from build123d import *

# Parameters (mm, degrees)
BOSS_EXTRUDE1_DEPTH = 50
BOSS_EXTRUDE2_DEPTH = 35
SKETCH4_R           = 2.2
CUT_EXTRUDE1_DEPTH  = 35
SKETCH5_R           = 4
CUT_EXTRUDE2_DEPTH  = 5
SKETCH6_R           = 4
CUT_EXTRUDE3_DEPTH  = 34
SKETCH7_R           = 4
SKETCH7_R_2         = 2.2
BOSS_EXTRUDE3_DEPTH = 8
SKETCH8_W           = 72
SKETCH8_H           = 52
BOSS_EXTRUDE4_DEPTH = 10
FILLET1_R           = 5
CUT_EXTRUDE5_DEPTH  = 28
SKETCH11_R          = 11.145843878
SKETCH11_R_2        = 4
BOSS_EXTRUDE6_DEPTH = 3


with BuildPart() as part:
    # Sketch1 → Boss-Extrude1 (new body)
    with BuildSketch(Plane(origin=(0, 0, 0), x_dir=(1, 0, 0), z_dir=(0, 1, 0))):
        with BuildLine():
            Line((-28, 23.5), (-28, -8.5))
            ThreePointArc((-28, -8.5), (-24.485281374, -16.985281374), (-16, -20.5))
            Line((-16, -20.5), (16, -20.5))
            ThreePointArc((16, -20.5), (24.485281374, -16.985281374), (28, -8.5))
            Line((28, -8.5), (28, 23.5))
            Line((28, 23.5), (36, 23.5))
            Line((36, 23.5), (36, 15.5))
            Line((36, 15.5), (36, -8.5))
            Line((36, -8.5), (36, -28.5))
            Line((36, -28.5), (16, -28.5))
            Line((16, -28.5), (-16, -28.5))
            Line((-16, -28.5), (-36, -28.5))
            Line((-36, -28.5), (-36, -8.5))
            Line((-36, -8.5), (-36, 15.5))
            Line((-36, 15.5), (-36, 23.5))
            Line((-36, 23.5), (-28, 23.5))
        make_face()
    extrude(amount=BOSS_EXTRUDE1_DEPTH)

    # Sketch3 → Boss-Extrude2 (add)
    with BuildSketch(Plane(origin=(0, 50, 0), x_dir=(1, 0, 0), z_dir=(0, 1, 0))):
        with BuildLine():
            Line((-36, 7.5), (-36, -8.5))
            Line((-36, -8.5), (-36, -28.5))
            Line((-36, -28.5), (-16, -28.5))
            Line((-16, -28.5), (16, -28.5))
            Line((16, -28.5), (36, -28.5))
            Line((36, -28.5), (36, -8.5))
            Line((36, -8.5), (36, 7.5))
            Line((36, 7.5), (28, 7.5))
            Line((28, 7.5), (21.128428342, 7.5))
            ThreePointArc((21.128428342, 7.5), (0.128823476, -13.371176524), (-20.87078139, 7.5))
            Line((-20.87078139, 7.5), (-28, 7.5))
            Line((-28, 7.5), (-36, 7.5))
        make_face()
    extrude(amount=BOSS_EXTRUDE2_DEPTH)

    # Sketch4 → Cut-Extrude1 (cut)
    with BuildSketch(Plane(origin=(0, 0, 20.5), x_dir=(-1, 0, 0), z_dir=(0, 0, -1))):
        with Locations((8, 33)):
            Circle(SKETCH4_R)
        with Locations((-8, 33)):
            Circle(SKETCH4_R)
        with Locations((-8, 17)):
            Circle(SKETCH4_R)
        with Locations((8, 17)):
            Circle(SKETCH4_R)
    extrude(amount=-CUT_EXTRUDE1_DEPTH, mode=Mode.SUBTRACT)

    # Sketch5 → Cut-Extrude2 (cut)
    with BuildSketch(Plane(origin=(0, 0, 20.5), x_dir=(-1, 0, 0), z_dir=(0, 0, -1))):
        with Locations((-8, 17)):
            Circle(SKETCH5_R)
        with Locations((8, 17)):
            Circle(SKETCH5_R)
    extrude(amount=-CUT_EXTRUDE2_DEPTH, mode=Mode.SUBTRACT)

    # Sketch6 → Cut-Extrude3 (cut)
    with BuildSketch(Plane.XY.offset(28.5)):
        with Locations((-8, 68)):
            Circle(SKETCH6_R)
        with Locations((8, 68)):
            Circle(SKETCH6_R)
    extrude(amount=-CUT_EXTRUDE3_DEPTH, mode=Mode.SUBTRACT)

    # Sketch7 → Boss-Extrude3 (add)
    # profile 1 of 2: a face of its own
    with BuildSketch(Plane.XY.offset(28.5)):
        with Locations((-8, 68)):
            Circle(SKETCH7_R)
        with Locations((-8, 68)):
            Circle(SKETCH7_R_2, mode=Mode.SUBTRACT)
    # profile 2 of 2: a face of its own
    with BuildSketch(Plane.XY.offset(28.5)):
        with Locations((8, 68)):
            Circle(SKETCH7_R)
        with Locations((8, 68)):
            Circle(SKETCH7_R_2, mode=Mode.SUBTRACT)
    extrude(amount=-BOSS_EXTRUDE3_DEPTH)

    # Sketch8 → Boss-Extrude4 (add)
    with BuildSketch(Plane.XZ):
        with Locations((0, 2.5)):
            Rectangle(SKETCH8_W, SKETCH8_H)
    extrude(amount=BOSS_EXTRUDE4_DEPTH)

    # Fillet1
    fillet1_edges = [part.edges().sort_by_distance(p)[0] for p in [
        (-36, -10, 2.5),
        (36, -10, 2.5),
        (32, 50, -23.5),
        (32, 50, -7.5),
        (-32, 50, -23.5),
        (-32, 50, -7.5),
    ]]
    fillet(fillet1_edges, radius=FILLET1_R)

    # Sketch9 → Cut-Extrude5 (cut)
    with BuildSketch(Plane.XZ.offset(10)):
        Polygon((-3.635500279, -0.98), (-7.399824034, -7.5), (7.657470986, -7.5), (3.893147231, -0.98), align=None)
        Polygon((7.657470986, -7.5), (-7.399824034, -7.5), (-3.635500279, -14.02), (3.893147231, -14.02), align=None)
    extrude(amount=-CUT_EXTRUDE5_DEPTH, mode=Mode.SUBTRACT)

    # Sketch11 → Boss-Extrude6 (add)
    with BuildSketch(Plane(origin=(0, -10, 0), x_dir=(-1, 0, 0), z_dir=(0, -1, 0))):
        with Locations((-0.128823476, 7.5)):
            Circle(SKETCH11_R)
        with Locations(Location((-0.128823476, 7.5, 0), (0, 0, 90))):
            Circle(SKETCH11_R_2, mode=Mode.SUBTRACT)
    extrude(amount=-BOSS_EXTRUDE6_DEPTH)


solid = part.part
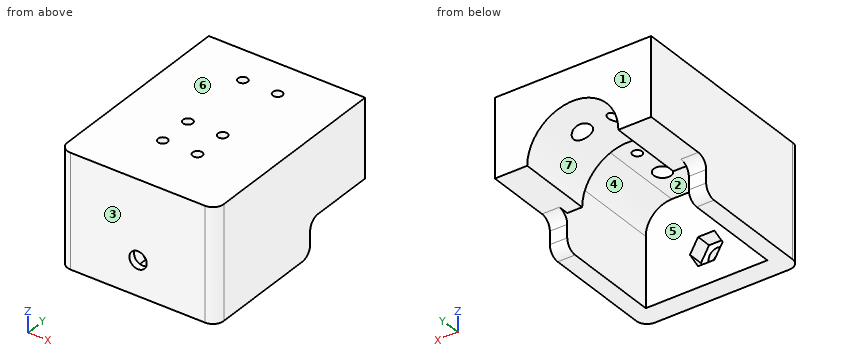
Design review of the part built by this model. Coordinates are the model's own, in mm. Face numbers are marked on the shaded views. A direction names the side the tool comes from. Give positions to 0.01 mm unless a question says otherwise; leave off trailing zeros. Loops run counter-clockwise (first coordinate to the right, second up) from the corner with the lowest first, then second, coordinate; pieces in that order, holes last. Notation, with made-up numbers: M 57,54.5 L 110,54.5 A17 cw 110,84.5 Z; hole C 45,-0.5 d8. An arc over 180 degrees is marked long. One line per question, with ' | ' between items. Start each with the question number.
1. Add section D-D (z = 11). Write out the cut boundary in (x, y), plus the area to 3 significant figures.
2. Add section C-C (x = -29.5). Write out the cut boundary in (y, z).
3. To check wall thickness, follow L1, parallel to Y at x = -8, z = 26.5; L2, parallel to X at y = 10, z = -16; L3, parallel to Y at x = 8, z = 22.15. State the ranges of each line that lie inside material, in increasing order.
4. The part is to be moulded in two halves that separate along Y. For the marked faces 1, 2, 3 and 4, say which applies: released by +Y, released by -Y, zero draft, split by the parting line, or undercut.
5. Add section A-A (y = 17). Write out the cut boundary in (x, z), plus the area to 3 significant figures.
6. Add section B-B (y = 28.5). Write out the cut boundary in (x, z), plus the area to 3 significant figures.
7. For the marked faces 5, 6 and 7, list the 3-axis set-ups (+Z, -Z, +X, -X, +Y, -Y) from which the entire face can be reached by the end or side of a thin tool; tool diameter is ignored.
8. Insertion check: P1, Ø16.5, axis at x = 29, y = 67.5, coming from the -Z side; P2, Ø1.5, axis at x = -15.5, y = 31, coming from the -Z side; P3, Ø7, axis at x = 0.13, z = -7.5, coming from the +Y side; P4, Ø13, axis at x = -7, z = -3, coming from the +Y side. Each pin has a flat end and moves straight along its axis. Give the tip position at first contact, or say it passes through.
Worked out:
1) outline: M -36,-5 A5 ccw -31,-10 L 31,-10 A5 ccw 36,-5 L 36,85 L 9.82,85 L 9.82,71.56 A4 cw 9.82,64.44 L 9.82,50 L 27.74,50 L 27.74,0 L -27.74,0 L -27.74,50 L -9.56,50 L -9.56,64.32 A4 cw -9.56,71.68 L -9.56,85 L -36,85 Z | area: 3,350 mm²
2) outline: M -10,-23.5 L 45,-23.5 A5 ccw 50,-18.5 L 50,-12.5 A5 cw 55,-7.5 L 85,-7.5 L 85,28.5 L -10,28.5 Z
3) L1: y = -10 to 14.8, 19.2 to 30.8, 35.2 to 65.8, 70.2 to 85 | L2: x = -36 to -28, 28 to 36 | L3: y = -10 to 13, 21 to 30.8, 35.2 to 65.8, 70.2 to 85
4) face 1: released by +Y | face 2: undercut | face 3: released by -Y | face 4: undercut
5) outline: M -36,-23.5 L -28,-23.5 L -28,8.5 A12 cw -16,20.5 L -12,20.5 L -12,25.5 L -10.2,25.5 L -10.2,28.5 L -36,28.5 Z; M -5.8,25.5 L -4,25.5 L -4,20.5 L 4,20.5 L 4,25.5 L 5.8,25.5 L 5.8,28.5 L -5.8,28.5 Z; M 10.2,25.5 L 12,25.5 L 12,20.5 L 16,20.5 A12 cw 28,8.5 L 28,-23.5 L 36,-23.5 L 36,28.5 L 10.2,28.5 Z | area: 1,240 mm²
6) outline: M -36,-23.5 L -28,-23.5 L -28,8.5 A12 cw -16,20.5 L 16,20.5 A12 cw 28,8.5 L 28,-23.5 L 36,-23.5 L 36,28.5 L -36,28.5 Z | area: 1,340 mm²
7) face 5: -Z | face 6: +Z, +X, -X, +Y, -Y | face 7: -Z, +Y
8) P1: stops at z = -7.5 | P2: stops at z = 20.5 | P3: passes through | P4: stops at y = 0
